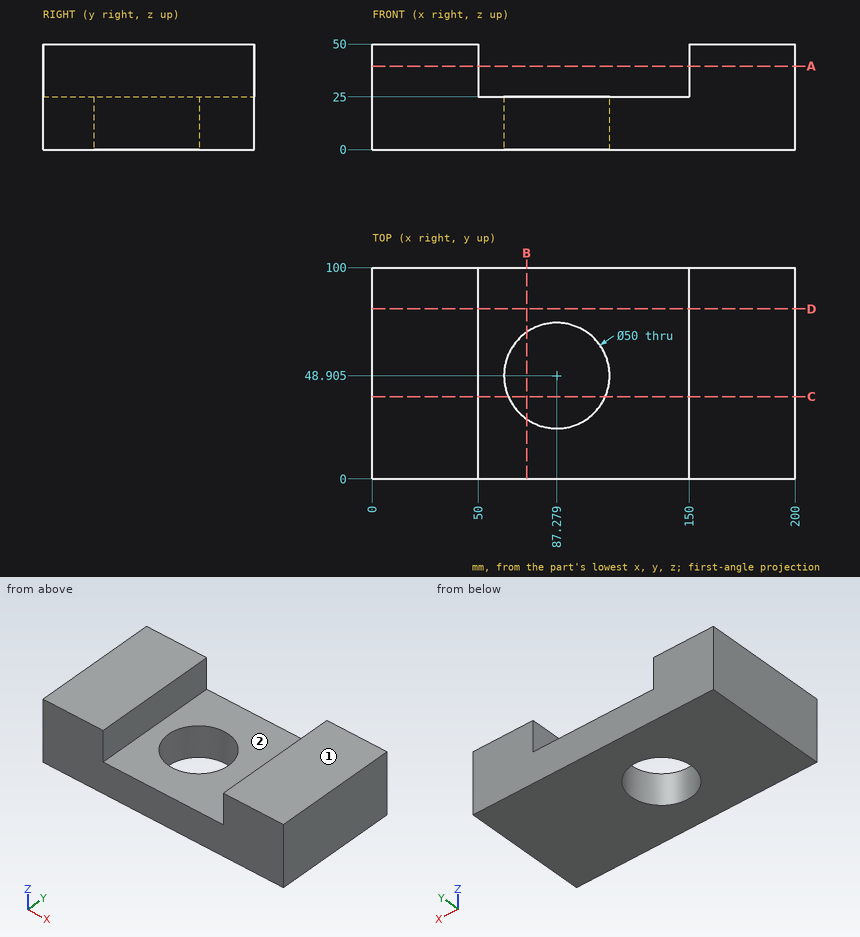
Here's the drawing with two shaded views (mm, measured from the low corner). I have some questions. A direction names the side the tool comes from. Coordinates: 2 decimals unless noted, no trailing zeros. Loops run counter-clockwise (first coordinate to the right, second up) from the corner with the lowest first, then second, coordinate; pieces in that order, holes last. Notation, with made-up numbers: (19, 36.25) - (34, 36.25) arc R6 ccw to (34, 43.25) - close; hole circle Ø11 at (71, 69.5). An arc over 180 degrees is marked (long way). Answer as CSV lines item,"result". Start each with the question number.
1) Suppose I cut it at A-A (z = 39.5). Please give me the cut outline in (x, y), plus the area to 3 significant figures.
2) Suppose I cut it at C-C (y = 39). Please give me the cut outline in (x, z) (1 decimal).
3) Which directions (+Z, -Z, +X, -X, +Y, -Y) give clear straight access to the entire face, cutting with the end or side of a thin tool? Please do the marked faces 1 and 2.
4) Suppose I cut it at B-B (x = 73). Please give me the cut outline in (y, z), plus the area to 3 significant figures.
5) I need wall thicknesses on line 1 (X direction, y = 43.5, z = 45.5); line 2 (Z direction, x = 140.5, y = 30.5); line 3 (Y direction, x = 80, z = 8). Which ranges of each line are inside material? Lowest first, please. Write a range as from..to.
6) Suppose I cut it at D-D (y = 80.5). Please give me the cut outline in (x, z).
7) For pin 1 (5 mm diameter, centred on y = 75, z = 31, fed in from -X); pin 2 (10 mm diameter, centred on x = 70, y = 34, fed in from +Z), each with a flat end and sliding along its axis, tell me the tip position at first contact or that it passes through.
Check result:
1,outline,"(0, 0) - (50, 0) - (50, 100) - (0, 100) - close; (150, 0) - (200, 0) - (200, 100) - (150, 100) - close"
1,area,"10,000 mm²"
2,outline,"(0, 0) - (64.3, 0) - (64.3, 25) - (50, 25) - (50, 50) - (0, 50) - close; (110.2, 0) - (200, 0) - (200, 50) - (150, 50) - (150, 25) - (110.2, 25) - close"
3,face 1,"+Z, +X, -X, +Y, -Y"
3,face 2,"+Z, +Y, -Y"
4,outline,"(0, 0) - (28.38, 0) - (28.38, 25) - (0, 25) - close; (69.43, 0) - (100, 0) - (100, 25) - (69.43, 25) - close"
4,area,"1,470 mm²"
5,line 1,"x = 0..50, 150..200"
5,line 2,"z = 0..25"
5,line 3,"y = 0..24.99, 72.82..100"
6,outline,"(0, 0) - (200, 0) - (200, 50) - (150, 50) - (150, 25) - (50, 25) - (50, 50) - (0, 50) - close"
7,pin 1,"stops at x = 0"
7,pin 2,"stops at z = 25"
